Work out the finished part from the listing and answer in its coordinate system (mm). A direction names the side the tool comes from. Coordinates: 2 decimals unless noted, no trailing zeros. Loops run counter-clockwise (first coordinate to the right, second up) from the corner with the lowest first, then second, coordinate; pieces in that order, holes last. Notation, with made-up numbers: (22.5, 30) -> (33.5, 30) arc R27 ccw to (33.5, 49) -> close; hole circle Ø10 at (75, 39.25). An arc over 180 degrees is marked (long way). Use a Markdown table: item, result.
Autodesk Inventor part; units mm, degrees
ref_plane "YZ Plane" through (0, 0, 0) normal (1, 0, 0) x (0, 1, 0)
ref_plane "XZ Plane" through (0, 0, 0) normal (0, 1, 0) x (-1, 0, 0)
ref_plane "XY Plane" through (0, 0, 0) normal (0, 0, 1) x (1, 0, 0)
sketch "Sketch1" plane through (0, 0, 0) normal (0, 1, 0) x (-1, 0, 0)
  line L0 (-23.54, 18.8125) -> (-23.54, -4.7733)
  line L1 (-23.54, 18.8125) -> (-23.54, 29.166)
  line L2 (-23.54, 29.166) -> (22.1671, 29.166)
  line L3 (22.1671, 29.166) -> (22.1671, -6.834)
  line L4 (18.6136, -6.834) -> (20.1065, -6.834)
  line L5 (22.1671, -4.7733) -> (22.1671, 18.8125)
  line L6 (-22.4793, 29.166) -> (21.1065, 29.166)
  line L7 (-23.54, 18.8125) -> (-23.54, -6.834)
  line L8 (-23.54, -6.834) -> (22.1671, -6.834)
  circle A0 centre (-0.6864, 8.0196) radius 16.05
  line L9 (-23.54, 29.166) -> (22.1671, 29.166)
  line L10 (22.1671, 29.166) -> (22.1671, 20.7196)
  line L11 (22.1671, 20.7196) -> (-23.54, 20.7196)
  line L12 (-23.54, 20.7196) -> (-23.54, 29.166)
  circle A1 centre (-0.6864, -15) radius 12.8668
  point P0 (0, 0)
  point P1 (7.98, -5.4895)
  point P2 (9.257, -6.834)
  point P3 (22.1671, 20.7196)
  point P4 (-23.54, 20.7196)
  point P5 (-23.54, -4.7733)
  point P6 (-10.6298, -6.834)
  point P7 (-9.3528, -5.4895)
  dimension "d0" = 0
  dimension "d1" = 32.1
  dimension "d2" = 0
  dimension "d3" = 0
extrude "Extrusion1" add sketch "Sketch1" along normal blind 50 contours L1 L11 A0 A1 L8 L7 L0 | L1 L2 L3 L11 A0 | L11 L3 L8 L4 A1 A0
sketch "Sketch5" plane through (0, 50, 0) normal (0, 1, 0) x (1, 0, 0)
  line L0 (23.54, -29.166) -> (23.54, 6.834)
  line L1 (23.54, 6.834) -> (21.54, 6.834)
  line L2 (21.54, 6.834) -> (21.54, -29.166)
  line L3 (21.54, -29.166) -> (23.54, -29.166)
  line L4 (23.54, -29.166) -> (23.54, 6.834)
  line L5 (-22.1671, 6.834) -> (-22.1671, -29.166)
  line L6 (-22.1671, 6.834) -> (-20.1671, 6.834)
  line L7 (-20.1671, 6.834) -> (-20.1671, -29.166)
  line L8 (-20.1671, -29.166) -> (-22.1671, -29.166)
  line L9 (-22.1671, -29.166) -> (-22.1671, 6.834)
  point P0 (0, 0)
  dimension "d16" = 2
  dimension "d17" = 2
extrude "Extrusion3" cut sketch "Sketch5" against normal blind 100
properties part number "SBR20_BearingBlock"
Q1. Determine the mould class of faces 1 (the flat face through (1, 25, 29.166)), 2 (the flat face through (-20.167, 25, 11)), 3 (the cylindrical face through (1.26, 24.65, 24.06)) for opening direction X: pulls with the +X half, pulls with the -X half, needs draft (parallel to the pull), parting line crosses it, or undercut.
Solved:
| item | result |
|---|---|
| face 1 | needs draft |
| face 2 | pulls with the -X half |
| face 3 | undercut |
Q2. Section B-B on x = -13.5 is taken. Determine the outline of the cut face in (y, z).
Solved:
| item | result |
|---|---|
| outline | (0, -6.83) -> (50, -6.83) -> (50, 0.51) -> (0, 0.51) -> close; (0, 15.53) -> (50, 15.53) -> (50, 29.17) -> (0, 29.17) -> close |
Q3. Section D-D on x = 3 is taken. Determine the outline of the cut face in (y, z).
Solved:
| item | result |
|---|---|
| outline | (0, 23.9) -> (50, 23.9) -> (50, 29.17) -> (0, 29.17) -> close |
Q4. Section A-A on z = -3.5 is taken. Determine the outline of the cut face in (x, y).
Solved:
| item | result |
|---|---|
| outline | (-20.17, 0) -> (-10.49, 0) -> (-10.49, 50) -> (-20.17, 50) -> close; (11.86, 0) -> (21.54, 0) -> (21.54, 50) -> (11.86, 50) -> close |
Q5. Section C-C on y = 13 is taken. Determine the outline of the cut face in (x, z), and give its area (3 significant figures).
Solved:
| item | result |
|---|---|
| outline | (-20.17, -6.83) -> (-9.26, -6.83) arc R12.87 cw to (-7.98, -5.49) arc R16.05 cw (long way) to (9.35, -5.49) arc R12.87 cw to (10.63, -6.83) -> (21.54, -6.83) -> (21.54, 29.17) -> (-20.17, 29.17) -> close |
| area | 697 mm² |
Q6. Consider line 1 (X direction, y = 38, z = 8); line 2 (X direction, y = 40, z = 5.5); line 3 (Z direction, x = -13, y = 29). Determine where each line is inside the solid, lowest interval first. Write a range as [from, to].
Solved:
| item | result |
|---|---|
| line 1 | [-20.17, -15.36], [16.74, 21.54] |
| line 2 | [-20.17, -15.16], [16.54, 21.54] |
| line 3 | [-6.83, -0.36], [16.4, 29.17] |
Q7. For faces 4 (the flat face through (1, 0, 27)), 5 (the cylindrical face through (10.024, 24.65, -6.148)), determine the directions among +Z, -Z, +X, -X, +Y, -Y from which every point of the face is accessible in a straight line to the end or side of a thin tool.
Solved:
| item | result |
|---|---|
| face 4 | +Z, -Z, +X, -X, -Y |
| face 5 | -Z, +Y, -Y |
